Design review of the part built by this model. Coordinates are the model's own, in mm. A direction names the side the tool comes from. Give positions to 0.01 mm unless a question says otherwise; leave off trailing zeros. Loops run counter-clockwise (first coordinate to the right, second up) from the corner with the lowest first, then second, coordinate; pieces in that order, holes last. Notation, with made-up numbers: (67.5, 35) -> (80.5, 35) arc R9 ccw to (80.5, 42) -> close; hole circle Ø11 at (76, 79.25). An arc over 180 degrees is marked (long way). Answer in a Markdown table with one row per item. Add a question column.
(1) For pin 1 (2 mm diameter, centred on x = 9.5, y = 10, fed in from -Z); pin 2 (1.5 mm diameter, centred on y = 8, z = 1, fed in from +X), all flat-tipped, find the tip position at first contact; note any pin that passes through.
(2) Draft analysis for pull direction Y (two halves, no side actions). For faces 1 (the cylindrical face through (-0.651, 11.957, 1.521)), 2 (the flat face through (12.542, 0.237, 1.479)), 3 (the cylindrical face through (-8.43, 24.98, 1.48)), state which applies: +Y half, -Y half, draft (parallel to the pull), parting line (faces both ways), or undercut.
(3) Consider section B-B on y = 7. Write out the cut boundary in (x, z), then the cut area to 3 significant figures.
(4) Consider section A-A on x = -9.5. Write out the cut boundary in (y, z), then the cut area to 3 significant figures.
(5) Consider section D-D on x = 0. Write out the cut boundary in (y, z).
(6) For line 1 (Y direction, x = -1, z = 1.6); line 2 (Y direction, x = 0, z = 1.1); line 3 (X direction, y = -19.5, z = 2.5), list the stretches that pass through material, from the lowest coordinate up.
(7) For faces 4 (the cylindrical face through (-2.63, -22.98, 1.48)), 5 (the flat face through (23.657, 20.626, 1.479)), list the 3-axis set-ups (+Z, -Z, +X, -X, +Y, -Y) from which the entire face can be reached by the end or side of a thin tool; tool diameter is ignored.
(8) Consider section C-C on z = 1.35. Write out the cut boundary in (x, y).
from build123d import *

# Parameters (mm, degrees)
SKETCH3_R           = 4
BOSS_EXTRUDE4_DEPTH = 3
SKETCH5_R           = 1.25
SKETCH5_R_2         = 5
CUT_EXTRUDE2_DEPTH  = 43.952434096
SKETCH6_R           = 1.75
CUT_EXTRUDE3_DEPTH  = 43.952434096


with BuildPart() as part:
    # Sketch3 → Boss-Extrude4 (new body)
    with BuildSketch(Plane.XY):
        with BuildLine():
            Line((-12.5, -15), (-12.5, 15))
            ThreePointArc((-12.5, 15), (-8.321357206, 25.088136105), (1.766778898, 29.266778898))
            Line((1.766778898, 29.266778898), (26.766778898, 29.266778898))
            ThreePointArc((26.766778898, 29.266778898), (31.28229963, 24.401899264), (26.095015576, 20.260756249))
            Line((26.095015576, 20.260756249), (21.150345096, 21.00253374))
            ThreePointArc((21.150345096, 21.00253374), (17.488439715, 20.116539535), (15.48452884, 16.926104149))
            Line((15.48452884, 16.926104149), (9.51547116, -16.926104149))
            ThreePointArc((9.51547116, -16.926104149), (-2.374739058, -26.049783342), (-12.5, -15))
        make_face()
        with Locations((-1.764648859, -19.076420455)):
            Circle(SKETCH3_R, mode=Mode.SUBTRACT)
    extrude(amount=BOSS_EXTRUDE4_DEPTH)

    # Sketch5 → Cut-Extrude2 (cut, through all)
    with BuildSketch(Plane.XY.offset(3)):
        with Locations((-9.5, 10)):
            Circle(SKETCH5_R)
        with Locations((9.5, 10)):
            Circle(SKETCH5_R)
        with Locations((0, 7)):
            Circle(SKETCH5_R_2)
    extrude(amount=-CUT_EXTRUDE2_DEPTH, mode=Mode.SUBTRACT)

    # Sketch6 → Cut-Extrude3 (cut, through all)
    with BuildSketch(Plane.XY.offset(3)):
        with Locations((26.766778898, 24.738714008)):
            Circle(SKETCH6_R)
    extrude(amount=-CUT_EXTRUDE3_DEPTH, mode=Mode.SUBTRACT)


solid = part.part
Values follow:
| question | item | result |
|---|---|---|
| 1 | pin 1 | through |
| 1 | pin 2 | x = 14.04 |
| 2 | face 1 | undercut |
| 2 | face 2 | -Y half |
| 2 | face 3 | +Y half |
| 3 | outline | (-12.5, 0) -> (-5, 0) -> (-5, 3) -> (-12.5, 3) -> close; (5, 0) -> (13.73, 0) -> (13.73, 3) -> (5, 3) -> close |
| 3 | area | 48.7 mm2 |
| 4 | outline | (-22.59, 0) -> (8.75, 0) -> (8.75, 3) -> (-22.59, 3) -> close; (11.25, 0) -> (23.75, 0) -> (23.75, 3) -> (11.25, 3) -> close |
| 4 | area | 132 mm2 |
| 5 | outline | (-26, 0) -> (-22.67, 0) -> (-22.67, 3) -> (-26, 3) -> close; (-15.49, 0) -> (2, 0) -> (2, 3) -> (-15.49, 3) -> close; (12, 0) -> (29.16, 0) -> (29.16, 3) -> (12, 3) -> close |
| 6 | line 1 | -26.08 to -23, -15.15 to 2.1, 11.9 to 29 |
| 6 | line 2 | -26 to -22.67, -15.49 to 2, 12 to 29.16 |
| 6 | line 3 | -11.55 to -5.74, 2.21 to 8.73 |
| 7 | face 4 | +Z, -Z |
| 7 | face 5 | +Z, -Z, -Y |
| 8 | outline | (-12.5, -15) arc R11.09 ccw to (9.52, -16.93) -> (15.48, 16.93) arc R5 cw to (21.15, 21) -> (26.1, 20.26) arc R4.53 ccw (long way) to (26.77, 29.27) -> (1.77, 29.27) arc R14.27 ccw to (-12.5, 15) -> close; hole circle Ø2.5 at (-9.5, 10); hole circle Ø8 at (-1.76, -19.08); hole circle Ø10 at (0, 7); hole circle Ø2.5 at (9.5, 10); hole circle Ø3.5 at (26.77, 24.74) |
